Verification items for the finished model (mm, model axes). A direction names the side the tool comes from. Coordinates: 2 decimals unless noted, no trailing zeros. Order: outer loops, then holes, each group sorted by start corner. A loop starts at its lowest first (then second) coordinate and runs counter-clockwise, first axis right, second up. Notation, with made-up numbers: M -5.75,-4 L 53.25,-4 A23 cw 53.25,20 Z; hole C 5.25,14 d11. An arc over 180 degrees is marked long. Return JSON: item names as keys, results as strings. Group by question number.
1. Set-up check for faces 5 (the flat face through (119, -36.024, 5)), 6 (the flat face through (98, -92.024, 5)): record each of +Z, -Z, +X, -X, +Y, -Y from which the full face is reachable in a straight line by a thin tool's end or side.
2. Section check C-C, the plane x = -92. Record the cut outline in (y, z) (1 decimal).
3. Material ranges on line 1 along Y through (x, z) = (119.5, 7); line 2 along X through (y, z) = (51.5, 1.5); line 3 along Y through (x, z) = (136, 5.5), recorded low to high.
4. Mould release check, pull along X, two halves, no side actions. Record for faces 1 (the flat face through (15, -39, 9.525)), 2 (the flat face through (224.714, -64, 5)), 3 (the cylindrical face through (-29.48, -91.28, 4.7)), 4 (the cylindrical face through (153.475, -59.218, 4.829)): +X half, -X half, draft (parallel to the pull), parting line (faces both ways), or undercut.
5. Section check A-A, the plane x = 147. Record the cut outline in (y, z) (3 decimals), plus the area to 3 significant figures.
6. Section check D-D, the plane x = -21.5. Record the cut outline in (y, z) (3 decimals), plus the area to 3 significant figures.
7. Section check B-B, the plane y = 56. Record the cut outline in (x, z) (3 decimals).
8. Gauge pin test, flat ends, axial feed: pin 1 (4 mm diameter, centred on x = 127.5, z = 3.5, fed in from +Y); pin 2 (4.5 mm diameter, centred on y = 17.98, z = 4.76, fed in from +X); pin 3 (2 mm diameter, centred on x = 3.5, y = -54, fed in from -Z); pin 4 (2 mm diameter, centred on y = -55, z = 7.5, fed in from -X). Record the tip position at first contact, or that the pin passes through.
```python
from build123d import *

# Parameters (mm, degrees)
RESSALTO_EXTRUS_O1_DEPTH = 9.525
ESBO_O3_R                = 16
CIRCULO_ROLAMENTO_DEPTH  = 10
ESBO_O6_R                = 2.5
CORTE_EXTRUS_O4_DEPTH    = 30
CORTE_EXTRUS_O6_DEPTH    = 10
ESBO_O10_R               = 2.78
CORTE_EXTRUS_O7_DEPTH    = 10
FILETE1_R                = 10
ESBO_O12_R               = 2.78
CORTE_EXTRUS_O8_DEPTH    = 10


with BuildPart() as part:
    # Esboço1 → Ressalto-extrusão1 (new body)
    with BuildSketch(Plane.XY):
        Polygon((-114.28595772, -92.023971813), (224.71404228, -92.023971813), (224.71404228, -36.023971813), (5.71404228, -36.023971813), (-54.28595772, 23.976028187), (-54.28595772, 92.976028187), (-114.28595772, 92.976028187), align=None)
    extrude(amount=RESSALTO_EXTRUS_O1_DEPTH)

    # Esboço3 → Circulo rolamento (cut)
    with BuildSketch(Plane.XY.offset(9.525)):
        with Locations((138.21404228, -64.023971813)):
            Circle(ESBO_O3_R)
    extrude(amount=-CIRCULO_ROLAMENTO_DEPTH, mode=Mode.SUBTRACT)

    # Esboço6 → Corte-extrusão4 (cut)
    with BuildSketch(Plane.ZY.offset(114.28595772)):
        with Locations(Location((4.7625, 67.976028187, 0), (0, 0, 270))):
            Circle(ESBO_O6_R)
        with Locations(Location((4.7625, 42.976028187, 0), (0, 0, 270))):
            Circle(ESBO_O6_R)
        with Locations(Location((4.7625, 17.976028187, 0), (0, 0, 270))):
            Circle(ESBO_O6_R)
    extrude(amount=-CORTE_EXTRUS_O4_DEPTH, mode=Mode.SUBTRACT)

    # Esboço9 → Corte-extrusão6 (cut)
    with BuildSketch(Plane.XY.offset(9.525)):
        Polygon((-29.841868762, -92.023971813), (-114.28595772, -7.579882856), (-114.28595772, -92.023971813), align=None)
    extrude(amount=-CORTE_EXTRUS_O6_DEPTH, mode=Mode.SUBTRACT)

    # Esboço10 → Corte-extrusão7 (cut)
    with BuildSketch(Plane.XY.offset(9.525)):
        with Locations((56.47404228, -50.023971813)):
            Circle(ESBO_O10_R)
        with Locations((56.47404228, -64.023971813)):
            Circle(ESBO_O10_R)
        with Locations((56.47404228, -78.023971813)):
            Circle(ESBO_O10_R)
    extrude(amount=-CORTE_EXTRUS_O7_DEPTH, mode=Mode.SUBTRACT)

    # Filete1
    filete1_edges = [part.edges().sort_by_distance(p)[0] for p in [
        (-54.28595772, 92.976028187, 4.7625),
        (-54.28595772, 23.976028187, 4.7625),
        (5.71404228, -36.023971813, 4.7625),
        (-29.841868762, -92.023971813, 4.7625),
    ]]
    fillet(filete1_edges, radius=FILETE1_R)

    # Esboço12 → Corte-extrusão8 (cut)
    with BuildSketch(Plane.XY.offset(9.525)):
        with Locations((219.95404228, -78.023971813)):
            Circle(ESBO_O12_R)
        with Locations((219.95404228, -64.023971813)):
            Circle(ESBO_O12_R)
        with Locations((219.95404228, -50.023971813)):
            Circle(ESBO_O12_R)
    extrude(amount=-CORTE_EXTRUS_O8_DEPTH, mode=Mode.SUBTRACT)


solid = part.part
```
Answers follow:
{
 "1": {"face 5": "+Z, -Z, +X, +Y", "face 6": "+Z, -Z, +X, -X, -Y"},
 "2": {"outline": "M -29.9,0 L 93,0 L 93,9.5 L -29.9,9.5 Z; hole C 18,4.8 d5; hole C 43,4.8 d5; hole C 68,4.8 d5"},
 "3": {"line 1": "-92.02 to -36.02", "line 2": "-114.29 to -54.29", "line 3": "-92.02 to -79.87, -48.18 to -36.02"},
 "4": {"face 1": "draft", "face 2": "+X half", "face 3": "-X half", "face 4": "undercut"},
 "5": {"outline": "M -92.024,0 L -77.396,0 L -77.396,9.525 L -92.024,9.525 Z; M -50.652,0 L -36.024,0 L -36.024,9.525 L -50.652,9.525 Z", "area": "279 mm^2"},
 "6": {"outline": "M -92.024,0 L -8.81,0 L -8.81,9.525 L -92.024,9.525 Z", "area": "793 mm^2"},
 "7": {"outline": "M -114.286,0 L -54.286,0 L -54.286,9.525 L -114.286,9.525 Z"},
 "8": {"pin 1": "y = -36.02", "pin 2": "x = -46.04", "pin 3": "z = 0", "pin 4": "x = -67.87"}
}
